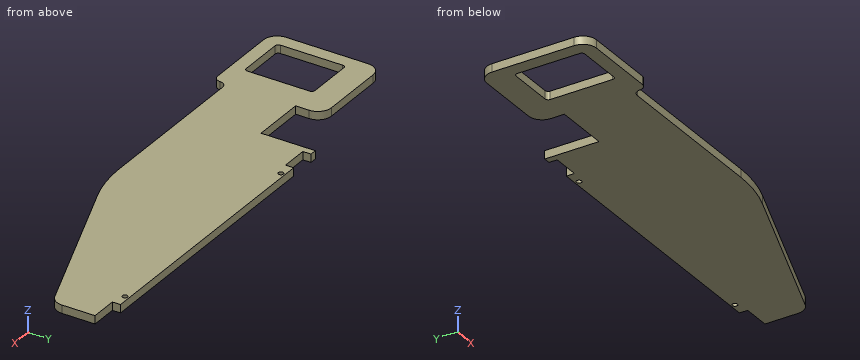
```python
from build123d import *

# Parameters (mm, degrees)
SKETCH1_R      = 1.86
EXTRUDE1_DEPTH = 6
FILLET1_R      = 10
FILLET2_R      = 5
FILLET4_R      = 100


with BuildPart() as part:
    # Sketch1 → Extrude1 (new body)
    with BuildSketch(Plane.XY):
        Polygon((58, 0), (58, -10), (-10, -10), (-10, 70.6), (58, 70.6), (58, 58.440884087), (58, 50.6), (98, 50.6), (98, 90.6), (103, 90.6), (103, 84.6), (123, 84.6), (123, 90.6), (323, 90.6), (323, 84.6), (343, 84.6), (343, 53.268621992), (200.6, 0), align=None)
        with Locations((313, 87.6)):
            Circle(SKETCH1_R, mode=Mode.SUBTRACT)
        with Locations((133, 87.6)):
            Circle(SKETCH1_R, mode=Mode.SUBTRACT)
        with BuildLine():
            Line((2.3, 50.6), (35.7, 50.6))
            ThreePointArc((35.7, 50.6), (37.326345597, 49.926345597), (38, 48.3))
            Line((38, 48.3), (38, 2.3))
            ThreePointArc((38, 2.3), (37.326345597, 0.673654403), (35.7, 0))
            Line((35.7, 0), (2.3, 0))
            ThreePointArc((2.3, 0), (0.673654403, 0.673654403), (0, 2.3))
            Line((0, 2.3), (0, 48.3))
            ThreePointArc((0, 48.3), (0.673654403, 49.926345597), (2.3, 50.6))
        make_face(mode=Mode.SUBTRACT)
    extrude(amount=EXTRUDE1_DEPTH)

    # Fillet1
    fillet1_edges = [part.edges().sort_by_distance(p)[0] for p in [
        (343, 53.268621992, 3),
        (-10, -10, 3),
        (-10, 70.6, 3),
        (58, 70.6, 3),
    ]]
    fillet(fillet1_edges, radius=FILLET1_R)

    # Fillet2
    fillet2_edges = [part.edges().sort_by_distance(p)[0] for p in [
        (58, 0, 3),
    ]]
    fillet(fillet2_edges, radius=FILLET2_R)
    fillet2_2_edges = [part.edges().sort_by_distance(p)[0] for p in [
        (58, -10, 3),
    ]]
    fillet(fillet2_2_edges, radius=FILLET2_R - 0.0001)  # a hair under: the kernel refuses the full size

    # Fillet4
    fillet4_edges = [part.edges().sort_by_distance(p)[0] for p in [
        (200.6, 0, 3),
    ]]
    fillet(fillet4_edges, radius=FILLET4_R)


solid = part.part
```
The model under review builds one solid part; all positions refer to its coordinate system, in mm. Round coordinates to 2 decimals unless told otherwise and drop trailing zeros. Write each loop counter-clockwise with the first axis right and the second up, starting at its lowest first coordinate (ties: lowest second). Pieces come first, ordered by that corner, then holes. Notation, with made-up numbers: (49, -18.75) - (95, -18.75) arc R15 cw to (95, -7.75) - close; hole circle Ø4 at (34, -40). An arc over 180 degrees is marked (long way). Use one line per item in the form item = value.
Q1. Consider section C-C (y = 78). State the section outline as (x, z) points.
Answer key:
outline = (98, 0) - (343, 0) - (343, 6) - (98, 6) - close
Q2. Consider section B-B (z = 4.2). State how many separate pieces and enclosed holes the cut face has, and give its area (3 significant figures).
Answer key:
separate_pieces = 1
enclosed_holes = 3
area = 23,600 mm2
Q3. For line 1 (X direction, y = 87.6, z = 4.75); line 2 (Y direction, x = 133, z = 1.65); line 3 (Y direction, x = 25, z = 1.2), list the stretches that pass through material, from the lowest coordinate up. Write a range as [from, to].
Answer key:
line_1 = [98, 103], [123, 131.14], [134.86, 311.14], [314.86, 323]
line_2 = [0, 85.74], [89.46, 90.6]
line_3 = [-10, 0], [50.6, 70.6]
Q4. Consider section A-A (y = 32). State the section outline as (x, z) points, and give its area (3 significant figures).
Answer key:
outline = (-10, 0) - (0, 0) - (0, 6) - (-10, 6) - close; (38, 0) - (286.14, 0) - (286.14, 6) - (38, 6) - close
area = 1,550 mm2
Q5. Insertion check: pin 1 Ø1.8 at (y, z) = (53, 2.5) entering from +X; pin 2 Ø1.8 at (x, z) = (330.5, 4.5) entering from +Y; pin 3 Ø3 at (y, z) = (88, 2.5) entering from +X. Each pin has a flat end and moves straight along its axis. Give the tip position at first contact, or say it passes through.
Answer key:
pin_1 = 340.76
pin_2 = 84.6
pin_3 = 323
